Autodesk Inventor part; units mm, degrees
ref_plane "_to_bjs_XY" through (27, 0, 0) normal (1, 0, 0) x (0, 0, -1)
ref_plane "_to_bjs_YZ" through (27, 0, 0) normal (0, 0, -1) x (0, 1, 0)
ref_plane "_to_bjs_ZX" through (27, 0, 0) normal (0, 1, 0) x (1, 0, 0)
sketch "Sketch_1" plane through (0, 0, 0) normal (0, 0, 1) x (1, 0, 0)
  line L0 (17, 0) -> (0, 0)
  line L1 (0, 0) -> (0, 17)
  line L2 (0, 17) -> (16.7, 17)
  arc A0 (16.7, 17) -> (17, 17.3) centre (16.7, 17.3) ccw
  line L3 (17, 17.3) -> (17, 0)
  line L4 (17, 0) -> (0, 0)
revolve "Revolution1" add sketch "Sketch_1" angle 360 about axis through (17, 0, 0) along (1, 0, 0)
sketch "Sketch_2" plane through (17, 0, 0) normal (1, 0, 0) x (0, 0, -1)
  line L0 (-21, 15.3297) -> (-21, -15.3297)
  arc A0 (-21, -15.3297) -> (-15.3297, -21) centre (0, 0) ccw
  line L1 (-15.3297, -21) -> (15.3297, -21)
  arc A1 (15.3297, -21) -> (21, -15.3297) centre (0, 0) ccw
  line L2 (21, -15.3297) -> (21, 15.3297)
  arc A2 (21, 15.3297) -> (15.3297, 21) centre (0, 0) ccw
  line L3 (15.3297, 21) -> (-15.3297, 21)
  arc A3 (-15.3297, 21) -> (-21, 15.3297) centre (0, 0) ccw
extrude "Extrusion1" add sketch "Sketch_2" along normal blind 10
sketch "_____4" plane through (0, 0, 0) normal (0, 0, 1) x (1, 0, 0)
  line L0 (54, 0) -> (-54, 0)
  line L1 (14.7, 17) -> (15, 16.7)
  line L2 (15, 16.7) -> (16.8, 16.7)
  arc A0 (16.8, 16.7) -> (17.3, 17.2) centre (16.8, 17.2) ccw
  line L3 (17.3, 17.2) -> (17.3, 19)
  line L4 (17.3, 19) -> (17, 19.3)
  line L5 (17, 19.3) -> (14.7, 17)
revolve "Revolution2" cut sketch "_____4" angle 360 about axis through (54, 0, 0) along (1, 0, 0)
sketch "_____5" plane through (0, 0, 0) normal (0, 0, 1) x (1, 0, 0)
  line L0 (54, 0) -> (-54, 0)
  line L1 (0, 17) -> (0, 16.85)
  line L2 (0, 16.85) -> (10, 16.85)
  line L3 (10, 16.85) -> (10.15, 17)
  line L4 (10.15, 17) -> (0, 17)
revolve "Revolution3" cut sketch "_____5" angle 360 about axis through (54, 0, 0) along (1, 0, 0)
sketch "Sketch_5" plane through (0, 0, 0) normal (0, 0, 1) x (1, 0, 0)
  line L0 (27, 0) -> (0, 0)
  line L1 (0, 0) -> (0, 10.5)
  line L2 (0, 10.5) -> (2, 10.5)
  line L3 (2, 10.5) -> (2, 7.25)
  line L4 (2, 7.25) -> (5, 7.25)
  line L5 (5, 7.25) -> (5, 5)
  line L6 (5, 5) -> (21, 5)
  line L7 (21, 5) -> (21, 7.25)
  line L8 (21, 7.25) -> (24, 7.25)
  line L9 (24, 7.25) -> (24, 10.5)
  line L10 (24, 10.5) -> (27, 11)
  line L11 (27, 11) -> (27, 0)
  line L12 (27, 0) -> (0, 0)
revolve "Revolution4" cut sketch "Sketch_5" angle 360 about axis through (27, 0, 0) along (1, 0, 0)
sketch "Sketch6" plane through (27, 0, 0) normal (1, 0, 0) x (0, 0, -1)
  point P0 (-14.8492, -14.8492)
hole "Hole1" at (27, -14.8492, 14.8492) direction (-1, 0, 0) diameter 4.5 depth 10 counterbore diameter 8 counterbore depth 4
pattern_linear "Rectangular Pattern1" count 2 spacing 29.6985 along (0, 0, -1) count 2 spacing 29.6985 along (0, 1, 0) of "Hole1"
sketch "Sketch_9" plane through (23, 0, 0) normal (1, 0, 0) x (0, 0, -1)
  line L0 (-21, 15.3297) -> (-21, -15.3297)
  arc A0 (-21, -15.3297) -> (-15.3297, -21) centre (0, 0) ccw
  line L1 (-15.3297, -21) -> (15.3297, -21)
  arc A1 (15.3297, -21) -> (21, -15.3297) centre (0, 0) ccw
  line L2 (21, -15.3297) -> (21, 15.3297)
  arc A2 (21, 15.3297) -> (15.3297, 21) centre (0, 0) ccw
  line L3 (15.3297, 21) -> (-15.3297, 21)
  arc A3 (-15.3297, 21) -> (-21, 15.3297) centre (0, 0) ccw
  line L4 (-20.95, 15.3134) -> (-20.95, -15.3134)
  arc A4 (-20.95, -15.3134) -> (-15.3134, -20.95) centre (0, 0) ccw
  line L5 (-15.3134, -20.95) -> (15.3134, -20.95)
  arc A5 (15.3134, -20.95) -> (20.95, -15.3134) centre (0, 0) ccw
  line L6 (20.95, -15.3134) -> (20.95, 15.3134)
  arc A6 (20.95, 15.3134) -> (15.3134, 20.95) centre (0, 0) ccw
  line L7 (15.3134, 20.95) -> (-15.3134, 20.95)
  arc A7 (-15.3134, 20.95) -> (-20.95, 15.3134) centre (0, 0) ccw
extrude "Extrusion2" cut sketch "Sketch_9" along normal mid plane 0.05
sketch "Sketch_10" plane through (27, 0, 0) normal (1, 0, 0) x (0, 0, -1)
  circle A0 centre (-15.9748, 5.8143) radius 3.5
  circle A1 centre (-15.9748, 5.8143) radius 3.1
extrude "Extrusion3" cut sketch "Sketch_10" against normal blind 1
pattern_linear "Rectangular Pattern2" count 2 spacing 24.0416 along (0, 0.4226, -0.9063) count 2 spacing 24.0416 along (0, -0.9063, -0.4226) of "Extrusion3"
sketch "Sketch_12" plane through (27, 0, 0) normal (1, 0, 0) x (0, 0, -1)
  line L0 (-17.4748, 4.9483) -> (-15.9748, 4.0823)
  line L1 (-15.9748, 4.0823) -> (-14.4748, 4.9483)
  line L2 (-14.4748, 4.9483) -> (-14.4748, 6.6804)
  line L3 (-14.4748, 6.6804) -> (-15.9748, 7.5464)
  line L4 (-15.9748, 7.5464) -> (-17.4748, 6.6804)
  line L5 (-17.4748, 6.6804) -> (-17.4748, 4.9483)
extrude "Extrusion4" cut sketch "Sketch_12" against normal blind 1
pattern_linear "Rectangular Pattern3" count 2 spacing 24.0416 along (0, 0.4226, -0.9063) count 2 spacing 24.0416 along (0, -0.9063, -0.4226) of "Extrusion4"
ref_plane "_to_bjs_XY" through (27, 0, 0) normal (1, 0, 0) x (0, 0, -1)
ref_plane "_to_bjs_YZ" through (27, 0, 0) normal (0, 0, -1) x (0, 1, 0)
ref_plane "_to_bjs_ZX" through (27, 0, 0) normal (0, 1, 0) x (1, 0, 0)
ref_plane "to_collar_XY" through (21, 0, 0) normal (-1, 0, 0) x (0, 0, -1)
ref_plane "to_collar_YZ" through (21, 0, 0) normal (0, 0, -1) x (0, -1, 0)
ref_plane "to_collar_ZX" through (21, 0, 0) normal (0, -1, 0) x (-1, 0, 0)
ref_plane "to_collar_2_XY" through (5, 0, 0) normal (1, 0, 0) x (0, 0, -1)
ref_plane "to_collar_2_YZ" through (5, 0, 0) normal (0, 0, -1) x (0, 1, 0)
ref_plane "to_collar_2_ZX" through (5, 0, 0) normal (0, 1, 0) x (1, 0, 0)
ref_plane "to_dummy_XY" through (0, 0, 0) normal (1, 0, 0) x (0, 0, -1)
ref_plane "to_dummy_YZ" through (0, 0, 0) normal (0, 0, -1) x (0, 1, 0)
ref_plane "to_dummy_ZX" through (0, 0, 0) normal (0, 1, 0) x (1, 0, 0)
properties part number "C-TFK10_b"
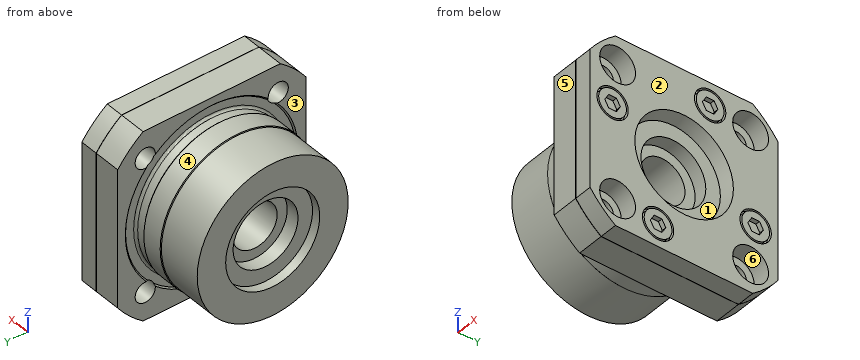
CAD build for the part. Positions are in the model's coordinates, mm. Face numbers are marked on the shaded views. A direction names the side the tool comes from. Round coordinates to 2 decimals unless told otherwise and drop trailing zeros. Order: outer loops, then holes, each group sorted by start corner. A loop starts at its lowest first (then second) coordinate and runs counter-clockwise, first axis right, second up.
Q1. Two-plate mould, pull along Y, no slides. Class the marked faces 4, 5 and 6: pulls with the +Y half, pulls with the -Y half, needs draft (parallel to the pull), parting line crosses it, or undercut.
Q2. Drop flat-ended pins along their axis: pin 1 (6 mm diameter, centred on y = -14.85, z = -14.85, fed in from +X); pin 2 (2 mm diameter, centred on x = 3.5, y = 12.5, fed in from -Z); pin 3 (6 mm diameter, centred on x = 3, y = 15, fed in from -Z). Give the stop position or say it passes through.
Q3. Wall check: L1, parallel to Z at x = 22.8, y = 0; L2, parallel to Z at x = 16.5, y = 0; L3, parallel to X at y = -16, z = -9.5. Give the ranges that are in metal, low to high.
Q4. Slice it at A-A (x = 6). Write the cut outline in (y, z).
Q5. Which spindle directions (+Z, -Z, +X, -X, +Y, -Y) get a long thin tool onto all of the face, cutting with end or side? Do the marked faces 1, 2 and 3. Say none if no direction does.
Q6. Slice it at B-B (z = -13.5). State how many separate pieces and enclosed holes the cut face has, and give its area (3 significant figures).
Results below:
1. face 4: parting line crosses it
1. face 5: pulls with the -Y half
1. face 6: undercut
2. pin 1: stops at x = 23
2. pin 2: stops at z = -12.32
2. pin 3: stops at z = -11.83
3. L1: z = -21 to -7.25, 7.25 to 21
3. L2: z = -16.7 to -5, 5 to 16.7
3. L3: x = 17.3 to 27
4. outline: circle Ø33.7 at (0, 0); hole circle Ø10 at (0, 0)
5. face 1: +X
5. face 2: +Z, -Z, +X, +Y, -Y
5. face 3: -X
6. separate pieces: 3
6. enclosed holes: 0
6. area: 658 mm2
